Geometry check sheet. Reference: the model listing, model coordinates, mm. Give positions to 0.01 mm unless a question says otherwise; leave off trailing zeros. Write each loop counter-clockwise with the first axis right and the second up, starting at its lowest first coordinate (ties: lowest second). Pieces come first, ordered by that corner, then holes. Notation, with made-up numbers: M -20,-12 L 7,-12 A23 cw 7,15 Z; hole C 5.5,18 d11. An arc over 180 degrees is marked long. One line per item, written item: value. Start each with the question number.
1. Scan lines: line 1 (Z direction, x = -2, y = 0); line 2 (Z direction, x = -0.5, y = -1.75); line 3 (X direction, y = -3.5, z = 114.5). Record each from-to range of solid material in increasing order.
2. Gauge pin test, flat ends, axial feed: pin 1 (4 mm diameter, centred on y = -3.5, z = 99, fed in from +X); pin 2 (1 mm diameter, centred on x = 2, z = 115, fed in from +Y). Record the tip position at first contact, or that the pin passes through.
3. Cross-section at B-B on x = 0.5. Count the separate pieces of the cut face and the enclosed holes in it, then the cut area to 3 significant figures.
4. Cross-section at A-A on z = 23. Record the cut outline in (x, y).
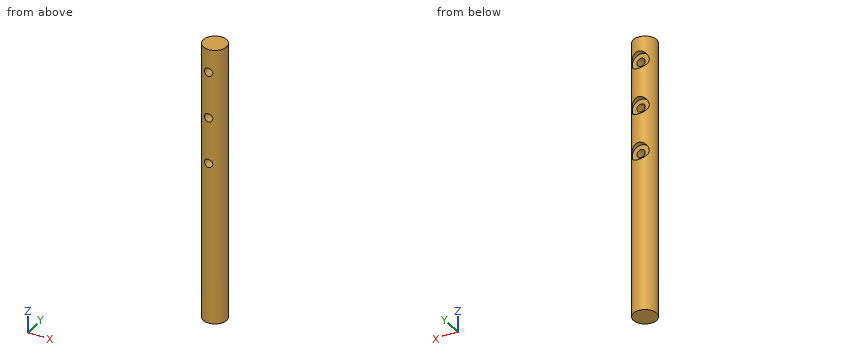
from build123d import *

# Parameters (mm, degrees)
SKETCH1_R                                           = 6.35
BOSS_EXTRUDE1_DEPTH                                 = 152.4
CBORE_FOR_8_BINDING_HEAD_MACHINE_SCREW1_D           = 4.4958
CBORE_FOR_8_BINDING_HEAD_MACHINE_SCREW1_CBORE_D     = 9.525
CBORE_FOR_8_BINDING_HEAD_MACHINE_SCREW1_CBORE_DEPTH = 2.667
CBORE_FOR_8_BINDING_HEAD_MACHINE_SC_2_D             = 4.4958
CBORE_FOR_8_BINDING_HEAD_MACHINE_SC_2_CBORE_D       = 9.525
CBORE_FOR_8_BINDING_HEAD_MACHINE_SC_2_CBORE_DEPTH   = 2.667
CBORE_FOR_8_BINDING_HEAD_MACHINE_SC_3_D             = 4.4958
CBORE_FOR_8_BINDING_HEAD_MACHINE_SC_3_CBORE_D       = 9.525
CBORE_FOR_8_BINDING_HEAD_MACHINE_SC_3_CBORE_DEPTH   = 2.667


with BuildPart() as part:
    # Sketch1 → Boss-Extrude1 (new body)
    with BuildSketch(Plane.XY):
        Circle(SKETCH1_R)
    extrude(amount=BOSS_EXTRUDE1_DEPTH)

    # CBORE for #8 Binding Head Machine Screw1 (through all)
    with Locations(Plane(origin=(-0.016915507, 6.34997747, 139.69710088), x_dir=(0.999996452, 0.002663859, 0), z_dir=(-0.002663859, 0.999996452, 0))):
        with Locations((0, 0)):
            CounterBoreHole(CBORE_FOR_8_BINDING_HEAD_MACHINE_SCREW1_D / 2, CBORE_FOR_8_BINDING_HEAD_MACHINE_SCREW1_CBORE_D / 2, CBORE_FOR_8_BINDING_HEAD_MACHINE_SCREW1_CBORE_DEPTH)

    # CBORE for _8 Binding Head Machine Sc 2 (through all)
    with Locations(Plane(origin=(-0.027009151, 6.349942559, 114.302510667), x_dir=(0.999990956, 0.004253, 0), z_dir=(-0.004253, 0.999990956, 0))):
        with Locations((0, 0)):
            CounterBoreHole(CBORE_FOR_8_BINDING_HEAD_MACHINE_SC_2_D / 2, CBORE_FOR_8_BINDING_HEAD_MACHINE_SC_2_CBORE_D / 2, CBORE_FOR_8_BINDING_HEAD_MACHINE_SC_2_CBORE_DEPTH)

    # CBORE for _8 Binding Head Machine Sc 3 (through all)
    with Locations(Plane(origin=(-0.003205304, 6.349999191, 88.90178774), x_dir=(0.999999872, 0.000505, 0), z_dir=(-0.000505, 0.999999872, 0))):
        with Locations((0, 0)):
            CounterBoreHole(CBORE_FOR_8_BINDING_HEAD_MACHINE_SC_3_D / 2, CBORE_FOR_8_BINDING_HEAD_MACHINE_SC_3_CBORE_D / 2, CBORE_FOR_8_BINDING_HEAD_MACHINE_SC_3_CBORE_DEPTH)


solid = part.part
Report:
1. line 1: z = 0 to 87.88, 89.93 to 113.28, 115.33 to 138.67, 140.72 to 152.4
1. line 2: z = 0 to 86.71, 91.09 to 112.11, 116.49 to 137.51, 141.89 to 152.4
1. line 3: x = -5.3 to -2.22, 2.25 to 5.3
2. pin 1: stops at x = 6.17
2. pin 2: stops at y = 3.69
3. separate pieces: 4
3. enclosed holes: 0
3. area: 1,720 mm^2
4. outline: C 0,0 d12.7
